Part print with two shaded views. Sizes in mm from the minimum x, y, z corner. A direction names the side the tool comes from. Round coordinates to 2 decimals unless told otherwise and drop trailing zeros. Order: outer loops, then holes, each group sorted by start corner. A loop starts at its lowest first (then second) coordinate and runs counter-clockwise, first axis right, second up. Notation, with made-up numbers: M 53.5,47 L 91.5,47 A11 cw 91.5,66 Z; hole C 19,80 d6. An arc over 180 degrees is marked long. Return JSON: item names as keys, results as strings. Group by question number.
Item 1: Pin check, flat tips, straight feed: pin 1 Ø0.9 at (x, z) = (0.5, 3.5) entering from -Y; pin 2 Ø1 at (x, z) = (2, 4) entering from -Y. Stop position of each tip, or through.
Item 2: Slice it at B-B on x = 2. Write the cut outline in (y, z).
Item 3: Which spindle directions (+Z, -Z, +X, -X, +Y, -Y) get a long thin tool onto all of the face, cutting with end or side? Do the marked faces 4 and 5. Say none if no direction does.
Item 4: Probe line 1 along Z through (x, y) = (5, 2.6) (1 decimal); line 2 along X through (y, z) = (4.2, 3.2) (1 decimal); line 3 along Y through (x, z) = (1.25, 1.35). List the from-to ranges inside material, lowest first.
Item 5: Pull direction Y, two halves, no side cores. Call the marked faces 1, 2 and 3: pulls with the +Y half, pulls with the -Y half, needs draft (parallel to the pull), parting line crosses it, or undercut.
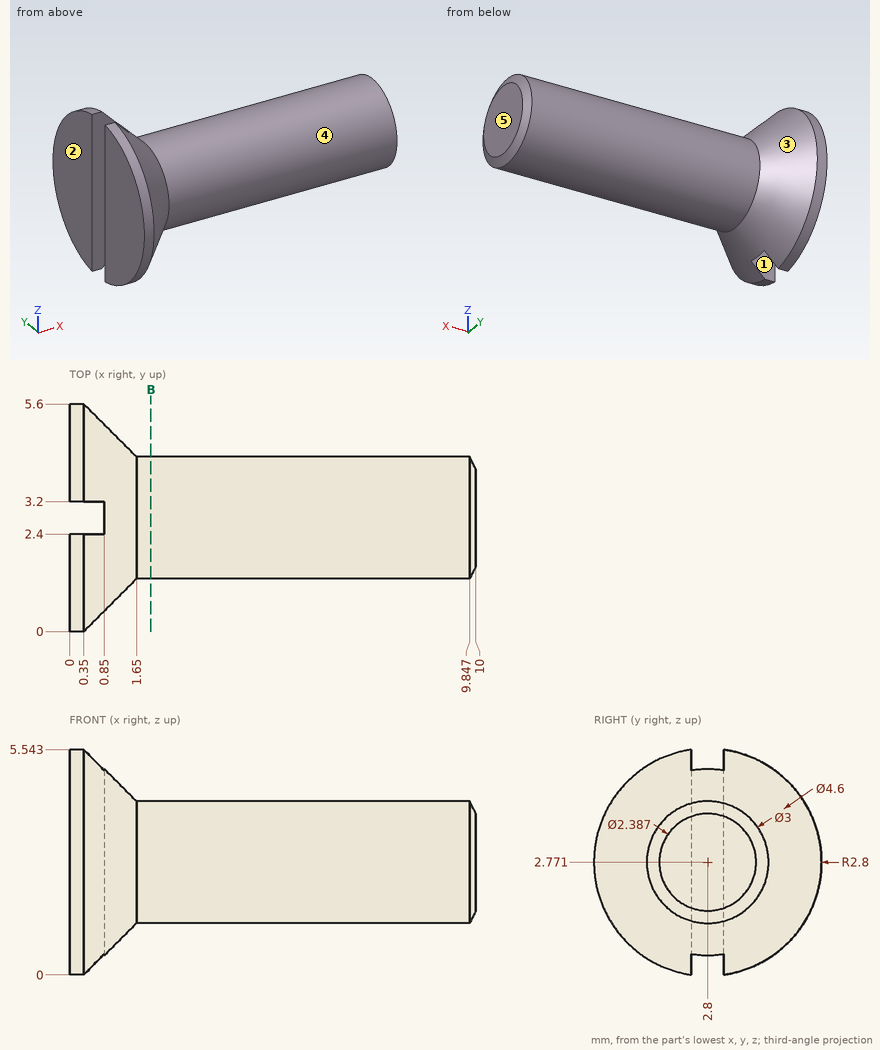
Output values:
{
 "1": {"pin 1": "y = 0.02", "pin 2": "y = 1.49"},
 "2": {"outline": "C 2.8,2.77 d3"},
 "3": {"face 4": "+X", "face 5": "+Z, -Z, +X, +Y, -Y"},
 "4": {"line 1": "1.3 to 4.3", "line 2": "0 to 9.9", "line 3": "1.54 to 4.06"},
 "5": {"face 1": "undercut", "face 2": "needs draft", "face 3": "parting line crosses it"}
}
